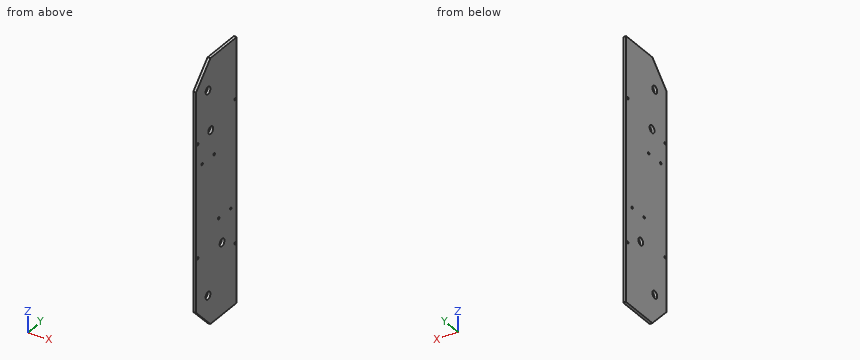
Autodesk Inventor part; units mm, degrees
ref_plane "YZ Plane" through (0, 0, 0) normal (1, 0, 0) x (0, 1, 0)
ref_plane "XZ Plane" through (0, 0, 0) normal (0, 1, 0) x (-1, 0, 0)
ref_plane "XY Plane" through (0, 0, 0) normal (0, 0, 1) x (1, 0, 0)
sketch "Sketch1" plane through (0, 0, 0) normal (1, 0, 0) x (0, 1, 0)
  line L0 (0, 0) -> (107.95, 0)
  line L1 (107.95, 0) -> (107.95, -444.5)
  line L2 (107.95, -444.5) -> (0, -444.5)
  line L3 (0, -444.5) -> (0, 0)
  circle A0 centre (31.75, -50.8) radius 6.3627
  circle A1 centre (31.75, -393.7) radius 6.3627
  circle A2 centre (92.6338, -165.5318) radius 1.5875
  circle A3 centre (76.6318, -165.5318) radius 1.5875
  circle A4 centre (15.3162, -278.9682) radius 1.5875
  circle A5 centre (31.3182, -278.9682) radius 1.5875
  dimension "d0" = 107.95
  dimension "d1" = 444.5
  dimension "d2" = 12.7254
  dimension "d3" = 31.75
  dimension "d4" = 50.8
  dimension "d5" = 50.8
  dimension "d22" = 165.5318
  dimension "d23" = 3.175
  dimension "d24" = 15.3162
  dimension "d25" = 3.175
  dimension "d26" = 16.002
  dimension "d27" = 165.5318
  dimension "d28" = 3.175
  dimension "d29" = 15.3162
  dimension "d30" = 165.5318
  dimension "d31" = 3.175
  dimension "d32" = 16.002
  dimension "d33" = 165.5318
extrude "Extrusion1" add sketch "Sketch1" along normal blind 4.7625 contours L0 L1 L2 L3 | A2 | A3 | A4 | A5
chamfer "Chamfer1" distance 38.1 angle 45 1 edges at (2.3813, 0, 0)
chamfer "Chamfer2" distance 38.1 angle 45 1 edges at (2.3813, 0, -444.5)
sketch "Sketch2" plane through (4.7625, 0, 0) normal (1, 0, 0) x (0, 0, -1)
  line L0 (444.5, 38.1) -> (406.4, 0)
  line L1 (444.5, 38.1) -> (444.5, 107.95)
  line L2 (444.5, 107.95) -> (0, 107.95)
  line L3 (0, 107.95) -> (0, 38.1)
  line L4 (38.1, 0) -> (0, 38.1)
  line L5 (38.1, 0) -> (406.4, 0)
  circle A0 centre (393.7, 31.75) radius 6.3627
  circle A1 centre (50.8, 31.75) radius 6.3627
  circle A2 centre (120.65, 38.989) radius 6.3627
  circle A3 centre (323.85, 68.961) radius 6.3627
  point P0 (0, 0)
  dimension "d14" = 12.7254
  dimension "d15" = 120.65
  dimension "d17" = 12.7254
  dimension "d19" = 120.65
  dimension "d78" = 38.989
  dimension "d79" = 38.989
extrude "Extrusion2" cut sketch "Sketch2" against normal blind 25.4 contours A2 | A3
sketch "Sketch6" plane through (4.7625, 0, 0) normal (1, 0, 0) x (0, 0, -1)
  circle A0 centre (120.65, 38.989) radius 6.3627
  circle A1 centre (323.85, 68.961) radius 6.3627
  line L0 (444.5, 38.1) -> (406.4, 0)
  line L1 (444.5, 38.1) -> (444.5, 107.95)
  line L2 (444.5, 107.95) -> (0, 107.95)
  line L3 (0, 107.95) -> (0, 38.1)
  line L4 (38.1, 0) -> (0, 38.1)
  line L5 (38.1, 0) -> (406.4, 0)
  circle A2 centre (393.7, 31.75) radius 6.3627
  circle A3 centre (50.8, 31.75) radius 6.3627
  point P0 (0, 0)
  point P1 (165.7604, 48.006)
  point P2 (165.7604, 16.002)
  point P3 (278.7396, 91.948)
  point P4 (278.7396, 59.944)
  dimension "d80" = 32.004
  dimension "d81" = 45.1104
  dimension "d82" = 45.1104
  dimension "d83" = 16.002
  dimension "d84" = 45.1104
  dimension "d85" = 45.1104
  dimension "d86" = 32.004
  dimension "d87" = 16.002
hole "Hole1" at (4.7625, 48.006, -165.7604) at (4.7625, 16.002, -165.7604) at (4.7625, 91.948, -278.7396) at (4.7625, 59.944, -278.7396) direction (-1, 0, 0) diameter 3.81 end through all
sketch "Sketch7" plane through (4.7625, 0, 0) normal (1, 0, 0) x (0, 0, -1)
  circle A0 centre (278.7396, 91.948) radius 1.905
  circle A1 centre (165.7604, 48.006) radius 1.905
  circle A2 centre (165.7604, 16.002) radius 1.905
  circle A3 centre (278.7396, 59.944) radius 1.905
  circle A4 centre (120.65, 38.989) radius 6.3627
  circle A5 centre (323.85, 68.961) radius 6.3627
  line L0 (444.5, 38.1) -> (406.4, 0)
  line L1 (444.5, 38.1) -> (444.5, 107.95)
  line L2 (444.5, 107.95) -> (0, 107.95)
  line L3 (0, 107.95) -> (0, 38.1)
  line L4 (38.1, 0) -> (0, 38.1)
  line L5 (38.1, 0) -> (406.4, 0)
  circle A6 centre (393.7, 31.75) radius 6.3627
  circle A7 centre (50.8, 31.75) radius 6.3627
  point P0 (0, 0)
  point P1 (101.6, 103.505)
  point P2 (342.9, 103.505)
  point P3 (127, 4.445)
  point P4 (317.5, 4.445)
  dimension "d95" = 4.445
  dimension "d96" = 4.445
  dimension "d97" = 4.445
  dimension "d98" = 4.445
  dimension "d99" = 101.6
  dimension "d100" = 101.6
  dimension "d101" = 127
  dimension "d102" = 127
hole "Hole2" at (4.7625, 103.505, -101.6) at (4.7625, 103.505, -342.9) at (4.7625, 4.445, -127) at (4.7625, 4.445, -317.5) direction (-1, 0, 0) diameter 3.81 depth 25.4 tip angle 118
equation "\"d19\" = d15"
properties part number "DriveTrain3.0"
Can you work these out from the model? Positions are in its coordinate system, mm. Round coordinates to 2 decimals unless told otherwise and drop trailing zeros. Loops run counter-clockwise (first coordinate to the right, second up) from the corner with the lowest first, then second, coordinate; pieces in that order, holes last. Notation, with made-up numbers: (76, -1.75) -> (121, -1.75) arc R7 cw to (121, 8.25) -> close; hole circle Ø6 at (20.5, 6). An arc over 180 degrees is marked (long way). One line per item, written item: value. Start each with the question number.
1. If we section it at B-B, the plane x = 2.2: Give the number of separate pieces and of enclosed holes in the cut face, then the cut area to 3 significant figures.
2. If we section it at A-A, the plane z = -323.85: Write out the boundary of the cut face in (x, y), then the cut area to 3 significant figures.
3. For pin 1 (2.5 mm diameter, centred on y = 48.01, z = -165.76, fed in from -X) (3 decimals), with a flat end and sliding along its axis, tell me the tip position at first contact or that it passes through.
4. If I drill on probe 1 along Y at (x, z) = (1.4, -393.7); probe 2 along Y at (x, z) = (1.65, -342.9); probe 3 along Z at (x, y) = (3.4, 31.75), over which ranges is the centre line in solid material (lowest first)?
Calculated:
1. separate pieces: 1
1. enclosed holes: 12
1. area: 45,900 mm²
2. outline: (0, 0) -> (4.76, 0) -> (4.76, 62.6) -> (0, 62.6) -> close; (0, 75.32) -> (4.76, 75.32) -> (4.76, 107.95) -> (0, 107.95) -> close
2. area: 454 mm²
3. pin 1: passes through
4. probe 1: y = 0 to 25.39, 38.11 to 107.95
4. probe 2: y = 0 to 101.6, 105.41 to 107.95
4. probe 3: z = -438.15 to -400.06, -387.34 to -57.16, -44.44 to -6.35
